Here's how the part is built. I have some questions about the finished solid (model axes, mm). Round coordinates to 2 decimals unless told otherwise and drop trailing zeros. Order: outer loops, then holes, each group sorted by start corner. A loop starts at its lowest first (then second) coordinate and runs counter-clockwise, first axis right, second up. Notation, with made-up numbers: M 36,-34.5 L 83,-34.5 A20 cw 83,-4.5 Z; hole C -8.75,-11.75 d11. An arc over 180 degrees is marked long. Write each question's results on one line, items separated by ' | '. Start each with the question number.
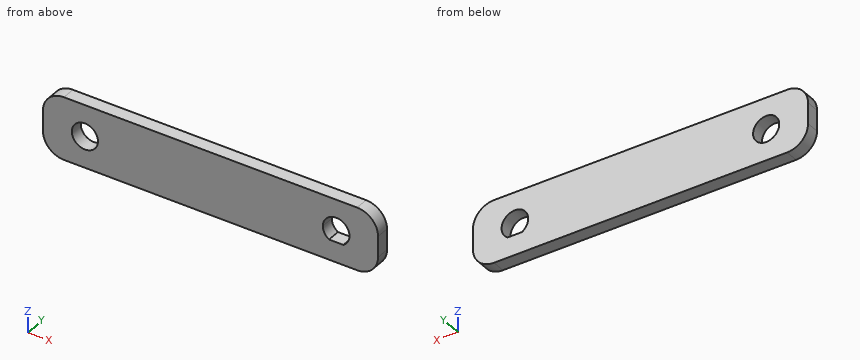
```python
from build123d import *

# Parameters (mm, degrees)
F0_R     = 3.125
F1_DEPTH = 3.175


with BuildPart() as f1:
    # F0 (on Front) → F1 (new body)
    with BuildSketch(Plane.XZ):
        with BuildLine():
            ThreePointArc((40, 2.5), (38.535534, 6.035534), (35, 7.5))
            Line((35, 7.5), (-35, 7.5))
            ThreePointArc((-35, 7.5), (-38.535534, 6.035534), (-40, 2.5))
            Line((-40, 2.5), (-40, -2.5))
            ThreePointArc((-40, -2.5), (-38.535534, -6.035534), (-35, -7.5))
            Line((-35, -7.5), (35, -7.5))
            ThreePointArc((35, -7.5), (38.535534, -6.035534), (40, -2.5))
            Line((40, -2.5), (40, 2.5))
        make_face()
        with Locations((-30, 0)):
            Circle(F0_R, mode=Mode.SUBTRACT)
        with BuildLine():
            ThreePointArc((28.289735, -2.674999), (27.212965, -1.525353), (26.820006, 0))
            ThreePointArc((26.820006, 0), (31.526083, 2.79582), (31.710265, -2.674999))
            Line((31.710265, -2.674999), (28.289735, -2.674999))
        make_face(mode=Mode.SUBTRACT)
    extrude(amount=F1_DEPTH)


solid = f1.part
```
(1) I want a section at A-A on x = -30. Write out the boundary of the cut face in (y, z) (3 decimals).
(2) I want a section at B-B on y = -1.3. Write out the boundary of the cut face in (x, z) (3 decimals).
(3) I want a section at C-C on z = 1.75. Write out the boundary of the cut face in (x, y) (3 decimals).
(4) I'm going to push flat-ended pins straight in: pin 1 Ø4 at (x, z) = (24, -5) entering from +Y; pin 2 Ø5 at (x, z) = (-30, 0) entering from -Y; pin 3 Ø1 at (y, z) = (-2, -5.5) entering from +X. Where does each tip first touch, or does it pass through?
(5) Please list where these lines run through material, in increasing order: line 1 (X direction, y = -0.9, z = -1.5); line 2 (Z direction, x = 30, y = -0.6) (3 decimals); line 3 (Z direction, x = 32, y = -0.9).
(6) I want a section at D-D on x = 30. Write out the boundary of the cut face in (y, z) (3 decimals).
Solutions:
1) outline: M -3.175,-7.5 L 0,-7.5 L 0,-3.125 L -3.175,-3.125 Z; M -3.175,3.125 L 0,3.125 L 0,7.5 L -3.175,7.5 Z
2) outline: M -40,-2.5 A5 ccw -35,-7.5 L 35,-7.5 A5 ccw 40,-2.5 L 40,2.5 A5 ccw 35,7.5 L -35,7.5 A5 ccw -40,2.5 Z; hole C -30,0 d6.25; hole M 26.82,0 A3.18 ccw 28.29,-2.675 L 31.71,-2.675 A3.18 ccw long Z
3) outline: M -40,-3.175 L -32.589,-3.175 L -32.589,0 L -40,0 Z; M -27.411,-3.175 L 27.341,-3.175 L 27.341,0 L -27.411,0 Z; M 32.659,-3.175 L 40,-3.175 L 40,0 L 32.659,0 Z
4) pin 1: y = 0 | pin 2: through | pin 3: x = 39.33
5) line 1: -40 to -32.74, -27.26 to 27.2, 32.8 to 40 | line 2: -7.5 to -2.675, 3.186 to 7.5 | line 3: -7.5 to -2.47, 2.48 to 7.5
6) outline: M -3.175,-7.5 L 0,-7.5 L 0,-2.675 L -3.175,-2.675 Z; M -3.175,3.186 L 0,3.186 L 0,7.5 L -3.175,7.5 Z
